from build123d import *

# Parameters (mm, degrees)
SKETCH1_W           = 40
SKETCH1_H           = 78
BOSS_EXTRUDE1_DEPTH = 22
SHELL1_T            = -1
CUT_EXTRUDE1_REACH  = 92.377
FILLET1_R           = 3
BOSS_EXTRUDE2_DEPTH = 13
CUT_EXTRUDE2_REACH  = 92.377
SKETCH4_W           = 10
SKETCH4_H           = 10
SKETCH6_W           = 1
SKETCH6_H           = 76
BOSS_EXTRUDE3_DEPTH = 15
SKETCH7_R           = 1.6
CUT_EXTRUDE3_DEPTH  = 15


with BuildPart() as part:
    # Sketch1 → Boss-Extrude1 (new body)
    with BuildSketch(Plane.XY):
        with Locations((20, 39)):
            Rectangle(SKETCH1_W, SKETCH1_H)
    extrude(amount=BOSS_EXTRUDE1_DEPTH)

    # Shell1
    shell1_openings = [part.faces().sort_by_distance(p)[0] for p in [
        (20, 39, 22),
    ]]
    offset(amount=SHELL1_T, openings=shell1_openings, kind=Kind.INTERSECTION)

    # Cut-Extrude1: up to this face of the body (flat: up to its plane)
    cut_extrude1_end = Plane(part.part.faces().sort_by_distance((0, 39, 11))[0])
    # Sketch2 → Cut-Extrude1 (cut, up to the picked face)
    with BuildSketch(Plane(origin=(40, 0, 0), x_dir=(0, 0, -1), z_dir=(1, 0, 0)), mode=Mode.PRIVATE) as cut_extrude1_sk1:
        Polygon((-22, 10), (-14, 10), (-14, 20), (-6, 20), (-6, 58), (-14, 58), (-14, 68), (-22, 68), align=None)
    cut_extrude1_tool1 = split(extrude(cut_extrude1_sk1.sketch, amount=-CUT_EXTRUDE1_REACH, mode=Mode.PRIVATE), bisect_by=cut_extrude1_end, keep=Keep.BOTH, mode=Mode.PRIVATE)
    add(cut_extrude1_tool1.solids().sort_by(Axis((40, 39, 14.833333), (-1, 0, 0)))[0], mode=Mode.SUBTRACT)

    # Fillet1
    fillet1_edges = [part.edges().sort_by_distance(p)[0] for p in [
        (0.5, 10, 22),
        (0.5, 68, 22),
        (0.5, 68, 14),
        (0.5, 58, 14),
        (0.5, 58, 6),
        (0.5, 20, 6),
        (0.5, 20, 14),
        (0.5, 10, 14),
        (39.5, 10, 22),
        (39.5, 68, 22),
        (39.5, 68, 14),
        (39.5, 58, 14),
        (39.5, 58, 6),
        (39.5, 20, 6),
        (39.5, 20, 14),
        (39.5, 10, 14),
    ]]
    fillet(fillet1_edges, radius=FILLET1_R)

    # Sketch3 → Boss-Extrude2 (add, symmetric)
    with BuildSketch(Plane(origin=(20, 0, 0), x_dir=(0, 0, -1), z_dir=(1, 0, 0))):
        with BuildLine():
            Line((-1, 1), (-19, 1))
            add(Edge.make_bspline(
                [(-19, 1), (-15.129811325, 9.249678545), (-5.265487128, 9.067042822)],
                knots=[0, 0, 0, 1, 1, 1], degree=2))
            Line((-5.265487128, 9.067042822), (-5.274742928, 8.567128499))
            add(Edge.make_bspline(
                [(-18.193150022, 1.5), (-16.753433037, 4.226674383), (-13.159011892, 6.996200729), (-8.728135169, 8.626895855), (-5.274742928, 8.567128499)],
                knots=[0.045482842, 0.045482842, 0.045482842, 0.403426776, 0.642056066, 1, 1, 1], degree=2))
            Line((-18.193150022, 1.5), (-1, 1.5))
            Line((-1, 1.5), (-1, 1))
        make_face()
        with BuildLine():
            Line((-5.274742928, 69.432871501), (-5.265487128, 68.932957178))
            add(Edge.make_bspline(
                [(-19, 77), (-15.129811325, 68.750321455), (-5.265487128, 68.932957178)],
                knots=[0, 0, 0, 1, 1, 1], degree=2))
            Line((-19, 77), (-1, 77))
            Line((-1, 77), (-1, 76.5))
            Line((-1, 76.5), (-18.193150022, 76.5))
            add(Edge.make_bspline(
                [(-18.193150022, 76.5), (-13.692591499, 70.12438977), (-5.274742928, 69.432871501)],
                knots=[0.057815428, 0.057815428, 0.057815428, 1, 1, 1], degree=2))
        make_face()
    extrude(amount=BOSS_EXTRUDE2_DEPTH, both=True)

    # Cut-Extrude2: up to this face of the body (flat: up to its plane)
    cut_extrude2_end = Plane(part.part.faces().sort_by_distance((20, 39, 1))[0])
    # Sketch4 → Cut-Extrude2 (cut, up to the picked face)
    with BuildSketch(Plane.XY.offset(22), mode=Mode.PRIVATE) as cut_extrude2_sk1:
        with Locations((20, 6)):
            Rectangle(SKETCH4_W, SKETCH4_H)
    cut_extrude2_tool1 = split(extrude(cut_extrude2_sk1.sketch, amount=-CUT_EXTRUDE2_REACH, mode=Mode.PRIVATE), bisect_by=cut_extrude2_end, keep=Keep.BOTH, mode=Mode.PRIVATE)
    # Sketch4 → Cut-Extrude2 (cut, up to the picked face)
    with BuildSketch(Plane.XY.offset(22), mode=Mode.PRIVATE) as cut_extrude2_sk2:
        with Locations((20, 72)):
            Rectangle(SKETCH4_W, SKETCH4_H)
    cut_extrude2_tool2 = split(extrude(cut_extrude2_sk2.sketch, amount=-CUT_EXTRUDE2_REACH, mode=Mode.PRIVATE), bisect_by=cut_extrude2_end, keep=Keep.BOTH, mode=Mode.PRIVATE)
    add(cut_extrude2_tool1.solids().sort_by(Axis((20, 6, 22), (0, 0, -1)))[0], mode=Mode.SUBTRACT)
    add(cut_extrude2_tool2.solids().sort_by(Axis((20, 72, 22), (0, 0, -1)))[0], mode=Mode.SUBTRACT)

    # Sketch6 → Boss-Extrude3 (add)
    with BuildSketch(Plane.XY.offset(1)):
        with Locations((20, 39)):
            Rectangle(SKETCH6_W, SKETCH6_H)
    extrude(amount=BOSS_EXTRUDE3_DEPTH)

    # Sketch7 → Cut-Extrude3 (cut)
    with BuildSketch(Plane.XY.offset(1)):
        with Locations((10.325, 11.175)):
            Circle(SKETCH7_R)
        with Locations((10.325, 66.825)):
            Circle(SKETCH7_R)
        with Locations((29.675, 11.175)):
            Circle(SKETCH7_R)
        with Locations((29.675, 66.825)):
            Circle(SKETCH7_R)
    extrude(amount=-CUT_EXTRUDE3_DEPTH, mode=Mode.SUBTRACT)


solid = part.part
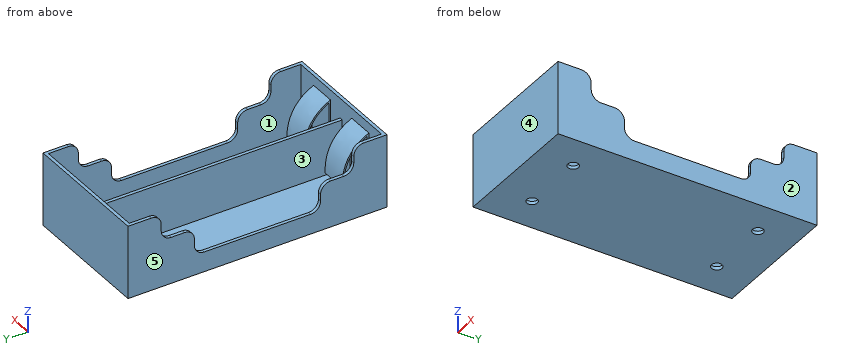
For this review, take the finished solid that the model builds, in its own axes (mm). Face numbers are marked on the shaded views. A direction names the side the tool comes from. Give positions to 0.01 mm unless a question says otherwise; leave off trailing zeros. Loops run counter-clockwise (first coordinate to the right, second up) from the corner with the lowest first, then second, coordinate; pieces in that order, holes last. Notation, with made-up numbers: (-26, 24) - (19, 24) arc R25 ccw to (19, 57) - close; hole circle Ø2 at (1, 83.5). An arc over 180 degrees is marked (long way). Write each question's results on one line, items separated by ' | '.
(1) For pin 1 Ø4 at (y, z) = (52.5, 10) entering from -X; pin 2 Ø2 at (x, y) = (5.5, 55.5) entering from +Z, all flat-tipped, find the tip position at first contact; note any pin that passes through.
Conclusion:
pin 1: x = 19.5 | pin 2: z = 1
(2) Take a section at D-D (z = 19.75). Give the boundary of the cut face in (x, y), then the cut area to 3 significant figures.
Conclusion:
outline: (0, 0) - (40, 0) - (40, 9.9) - (39, 9.9) - (39, 1) - (1, 1) - (1, 9.9) - (0, 9.9) - close; (0, 68.1) - (1, 68.1) - (1, 77) - (39, 77) - (39, 68.1) - (40, 68.1) - (40, 78) - (0, 78) - close | area: 116 mm^2
(3) For the marked faces 1 and 2, list the 3-axis set-ups (+Z, -Z, +X, -X, +Y, -Y) from which the entire face can be reached by the end or side of a thin tool; tool diameter is ignored.
Conclusion:
face 1: +Z | face 2: +Z, -Z, +X, +Y, -Y
(4) For line 1 along X through (y, z) = (10, 12.25); line 2 along Y through (x, z) = (18.5, 5.25); line 3 along Y through (x, z) = (10.5, 10.75), list the stretches that pass through material, from the lowest coordinate up.
Conclusion:
line 1: 0 to 1, 19.5 to 20.5, 39 to 40 | line 2: 0 to 1, 77 to 78 | line 3: 0 to 1.5, 7.86 to 8.39, 69.61 to 70.64, 76.5 to 78
(5) Take a section at B-B (y = 33.5). Give the boundary of the cut face in (x, z).
Conclusion:
outline: (0, 0) - (40, 0) - (40, 6) - (39, 6) - (39, 1) - (20.5, 1) - (20.5, 16) - (19.5, 16) - (19.5, 1) - (1, 1) - (1, 6) - (0, 6) - close
(6) Take a section at C-C (x = 4). Give the boundary of the cut face in (y, z).
Conclusion:
outline: (0, 0) - (78, 0) - (78, 22) - (77, 22) - (77, 1) - (1, 1) - (1, 22) - (0, 22) - close
(7) Take a section at A-A (z = 2.75). Give the boundary of the cut face in (x, y), then the cut area to 3 significant figures.
Conclusion:
outline: (0, 0) - (40, 0) - (40, 78) - (0, 78) - close; hole (1, 1) - (7, 1) - (7, 1.5) - (15, 1.5) - (15, 1) - (19.5, 1) - (19.5, 77) - (15, 77) - (15, 76.5) - (7, 76.5) - (7, 77) - (1, 77) - close; hole (20.5, 1) - (25, 1) - (25, 1.5) - (33, 1.5) - (33, 1) - (39, 1) - (39, 77) - (33, 77) - (33, 76.5) - (25, 76.5) - (25, 77) - (20.5, 77) - close | area: 324 mm^2
(8) Draft analysis for pull direction X (two halves, no side actions). For the marked faces 3, 4 and 5, state which applies: +X half, -X half, draft (parallel to the pull), parting line (faces both ways), or undercut.
Conclusion:
face 3: undercut | face 4: draft | face 5: -X half
